Source: three-view drawing plus pictorial views. Frame: mm from the lowest corner of the part. Coordinates: 2 decimals unless noted, no trailing zeros. Write each loop counter-clockwise with the first axis right and the second up, starting at its lowest first coordinate (ties: lowest second). Pieces come first, ordered by that corner, then holes. Notation, with made-up numbers: (59, -40) - (72, -40) arc R20 ccw to (72, -28) - close; hole circle Ø9 at (-38, 1.25). An arc over 180 degrees is marked (long way). One line per item, written item: value.
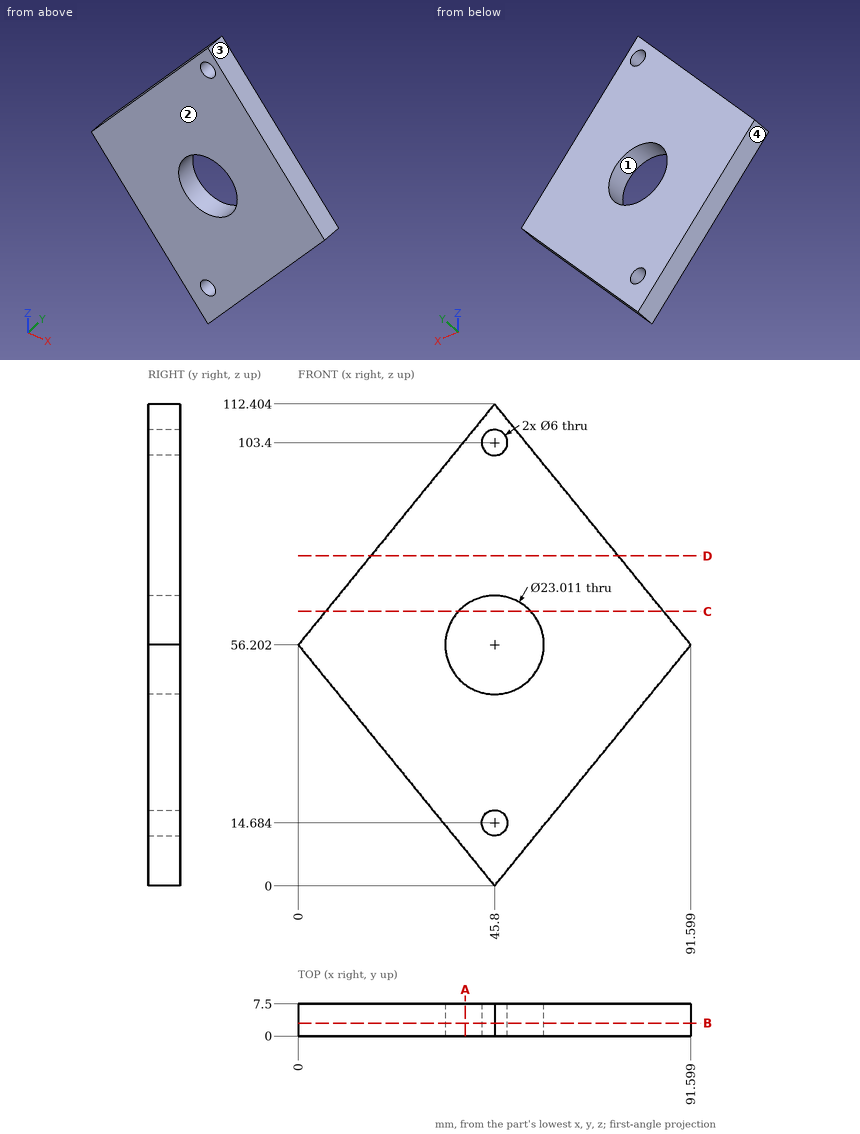
1) Material intervals for line 1 (X direction, y = 4, z = 54.5) (1 decimal); line 2 (X direction, y = 4.75, z = 64) (1 decimal); line 3 (X direction, y = 6.5, z = 86.5), sorted ascending.
Values found:
line 1: 1.4 to 34.4, 57.2 to 90.2
line 2: 6.4 to 37.3, 54.3 to 85.2
line 3: 24.69 to 66.91
2) Section query D-D on z = 77. Output: boundary loops of the cut face in (x, y), then the cut area to 3 significant figures.
Values found:
outline: (16.95, 0) - (74.65, 0) - (74.65, 7.5) - (16.95, 7.5) - close
area: 433 mm2
3) Section query B-B on y = 3. Output: boundary loops of the cut face in (x, z) (1 decimal).
Values found:
outline: (0, 56.2) - (45.8, 0) - (91.6, 56.2) - (45.8, 112.4) - close; hole circle Ø23 at (45.8, 56.2); hole circle Ø6 at (45.8, 14.7); hole circle Ø6 at (45.8, 103.4)
4) Section query A-A on x = 39. Output: boundary loops of the cut face in (y, z).
Values found:
outline: (0, 8.34) - (7.5, 8.34) - (7.5, 46.92) - (0, 46.92) - close; (0, 65.48) - (7.5, 65.48) - (7.5, 104.06) - (0, 104.06) - close
5) Section query C-C on z = 64. Output: boundary loops of the cut face in (x, y) (1 decimal), then the cut area to 3 significant figures.
Values found:
outline: (6.4, 0) - (37.3, 0) - (37.3, 7.5) - (6.4, 7.5) - close; (54.3, 0) - (85.2, 0) - (85.2, 7.5) - (54.3, 7.5) - close
area: 465 mm2
6) Contact query for flat-ended pins moving along their axis: P1, Ø14, axis at x = 45.8, z = 56.2, coming from the -Y side; P2, Ø2, axis at x = 40.5, y = 4, coming from the +Z side; P3, Ø1, axis at x = 14.5, y = 5.5, coming from the -Z side (1 decimal); P4, Ø1.5, axis at y = 3, z = 79.5, coming from the +X side (1 decimal). Output: stop coordinate, or through.
Values found:
P1: through
P2: z = 107.13
P3: z = 37.8
P4: x = 73.2
7) Draft query along Z for the marked faces 1, 2, 3 and 4. Return one class per face: released by +Z, released by -Z, zero draft, split by the parting line, or undercut.
Values found:
face 1: undercut
face 2: zero draft
face 3: released by +Z
face 4: released by -Z
